Geometry: final body of the model. Coordinates: model frame, mm. A direction names the side the tool comes from. Give positions to 0.01 mm unless a question says otherwise; leave off trailing zeros. Write each loop counter-clockwise with the first axis right and the second up, starting at its lowest first coordinate (ties: lowest second). Pieces come first, ordered by that corner, then holes. Notation, with made-up numbers: (78.5, 14) - (111.5, 14) arc R30 cw to (111.5, 41) - close; hole circle Ø1 at (-21.5, 61.5). An arc over 180 degrees is marked (long way). Return JSON: item names as keys, results as strings.
Autodesk Fusion 360 part; units mm, degrees
sketch "Sketch1" plane through (0, 0, 0) normal (0, 1, 0) x (1, 0, 0)
  circle A0 centre (0, 0) radius 13.85
  dimension "d1" = 27.7
extrude "Extrude1" add sketch "Sketch1" along normal blind 38
sketch "Sketch2" plane through (0, 38, 0) normal (0, 1, 0) x (-1, 0, 0)
  circle A0 centre (0, 0) radius 13.85
  circle A1 centre (0, 0) radius 5
  dimension "d4" = 10
extrude "Extrude2" add sketch "Sketch2" along normal blind 2.6 contours A1
sketch "Sketch3" plane through (0, 40.6, 0) normal (0, 1, 0) x (-1, 0, 0)
  circle A0 centre (0, 0) radius 5
  circle A1 centre (0, 0) radius 1.15
  dimension "d7" = 2.3
extrude "Extrude3" add sketch "Sketch3" along normal blind 14.55 contours A1
sketch "Sketch4" plane through (0, 0, 0) normal (0, -1, 0) x (1, 0, 0)
  circle A0 centre (0, 0) radius 13.85
  circle A1 centre (0, 0) radius 5
  dimension "d10" = 10
extrude "Extrude4" cut sketch "Sketch4" against normal blind 2.2
fillet "Fillet1" radius 1 1 edges at (-12.9127, 38, 5.0084)
fillet "Fillet2" radius 0.5 1 edges at (1.0722, 55.15, -0.4159)
fillet "Fillet3" radius 0.1 2 edges at (-12.9127, 2.2, 5.0084) (-4.6616, 0, -1.8081)
Q1. Pin query (flat end, axial travel): P1, Ø1.5, axis at x = 6, z = 4, coming from the +Y side; P2, Ø5, axis at x = 4, z = 0.5, coming from the +Y side; P3, Ø5, axis at x = -8.5, z = 1.5, coming from the -Y side. Return the tip coordinate at first contact, or that it passes through.
Answer key:
{"P1": "stops at y = 38", "P2": "stops at y = 40.6", "P3": "stops at y = 2.2"}
Q2. Section query B-B, the plane x = 0. Return the cut outline in (y, z).
Answer key:
{"outline": "(0, -4.9) arc R0.1 ccw to (0.1, -5) - (2.2, -5) - (2.2, -13.75) arc R0.1 ccw to (2.3, -13.85) - (37, -13.85) arc R1 ccw to (38, -12.85) - (38, -5) - (40.6, -5) - (40.6, -1.15) - (54.65, -1.15) arc R0.5 ccw to (55.15, -0.65) - (55.15, 0.65) arc R0.5 ccw to (54.65, 1.15) - (40.6, 1.15) - (40.6, 5) - (38, 5) - (38, 12.85) arc R1 ccw to (37, 13.85) - (2.3, 13.85) arc R0.1 ccw to (2.2, 13.75) - (2.2, 5) - (0.1, 5) arc R0.1 ccw to (0, 4.9) - close"}
Q3. Section query A-A, the plane z = 0. Return the cut outline in (x, y), plus the area to 3 significant figures.
Answer key:
{"outline": "(-13.85, 2.3) arc R0.1 ccw to (-13.75, 2.2) - (-5, 2.2) - (-5, 0.1) arc R0.1 ccw to (-4.9, 0) - (4.9, 0) arc R0.1 ccw to (5, 0.1) - (5, 2.2) - (13.75, 2.2) arc R0.1 ccw to (13.85, 2.3) - (13.85, 37) arc R1 ccw to (12.85, 38) - (5, 38) - (5, 40.6) - (1.15, 40.6) - (1.15, 54.65) arc R0.5 ccw to (0.65, 55.15) - (-0.65, 55.15) arc R0.5 ccw to (-1.15, 54.65) - (-1.15, 40.6) - (-5, 40.6) - (-5, 38) - (-12.85, 38) arc R1 ccw to (-13.85, 37) - close", "area": "1,070 mm^2"}
Q4. Material intervals for probe 1 along Y at (x, z) = (6.5, 1.5); probe 2 along Z at (x, y) = (-1.75, 3.5); probe 3 along X at (y, z) = (8.5, 12), sorted ascending. Write a range as [from, to].
Answer key:
{"probe 1": "y = [2.2, 38]", "probe 2": "z = [-13.74, 13.74]", "probe 3": "x = [-6.92, 6.92]"}
Q5. Section query C-C, the plane y = 26. Return the cut outline in (x, z), plus the area to 3 significant figures.
Answer key:
{"outline": "circle Ø27.7 at (0, 0)", "area": "603 mm^2"}
Q6. Set-up query: faces 1 (the flat face through (0, 2.2, -6)), 2 (the cylindrical face through (0.91, 47.53, 0.7)), 3 (the cylindrical face through (13.21, 19.41, 4.16)). Return all of +Z, -Z, +X, -X, +Y, -Y with unobstructed straight access to the full face (end or side cutting, diameter ignored); none if empty.
Answer key:
{"face 1": "-Y", "face 2": "+Y", "face 3": "+Y, -Y"}
